Could you check a few things on this model? Use its own coordinates, in mm. Face numbers are marked on the shaded views. Coordinates: 2 decimals unless noted, no trailing zeros. Order: outer loops, then holes, each group sorted by start corner. A loop starts at its lowest first (then second) coordinate and runs counter-clockwise, first axis right, second up. Notation, with made-up numbers: (9.5, 43) - (23.5, 43) arc R14 ccw to (23.5, 69) - close; hole circle Ø8 at (24, -6.5). An arc over 180 degrees is marked (long way). One line per item, written item: value.
from build123d import *

# Parameters (mm, degrees)
F2_DEPTH = 12.7
F1_R     = 6.35
F3_DEPTH = 25.4


with BuildPart() as f2:
    # F0 (on Front) → F2 (new body)
    with BuildSketch(Plane.XZ):
        with BuildLine():
            ThreePointArc((-28.403627, 25.393778), (-36.341802, -10.856114), (-9.82124, -36.812406))
            Line((-9.82124, -36.812406), (-3.273747, -12.270802))
            ThreePointArc((-3.273747, -12.270802), (17.211851, -4.772017), (20.836528, 16.739681))
            ThreePointArc((20.836528, 16.739681), (-1.537184, 33.848118), (-28.403627, 25.393778))
        make_face()
    extrude(amount=F2_DEPTH)

    # F1 (on face) → F3 (cut)
    with BuildSketch(Plane.XZ):
        Circle(F1_R)
    extrude(amount=F3_DEPTH, mode=Mode.SUBTRACT)


solid = f2.part
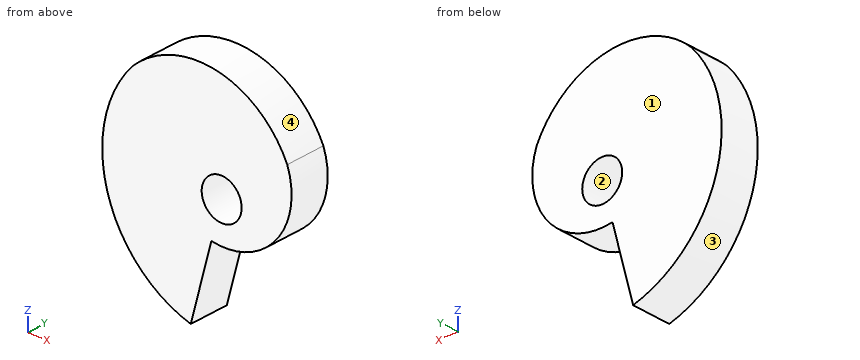
Item 1: I want a section at D-D on x = -20. Please give me the cut outline in (y, z).
Conclusion:
outline: (-12.7, -32.33) - (0, -32.33) - (0, 31.33) - (-12.7, 31.33) - close
Item 2: I want a section at A-A on x = 0. Please give me the cut outline in (y, z).
Conclusion:
outline: (-12.7, -12.6) - (0, -12.6) - (0, -6.35) - (-12.7, -6.35) - close; (-12.7, 6.35) - (0, 6.35) - (0, 33.54) - (-12.7, 33.54) - close
Item 3: If I drill on probe 1 along Z at (x, y) = (0, -9.5); probe 2 along X at (y, z) = (-2.5, 0); probe 3 along Z at (x, y) = (5, -3.5), over which ranges is the centre line in solid material (lowest first)?
Conclusion:
probe 1: -12.6 to -6.35, 6.35 to 33.54
probe 2: -37.94 to -6.35, 6.35 to 20.22
probe 3: -12.14 to -3.91, 3.91 to 31.93
Item 4: Thinking about a two-plate mould opening in X: for the marked faces 1, 2, 3 and 4, which applies, pulls with the +X half, pulls with the -X half, needs draft (parallel to the pull), parting line crosses it, or undercut?
Conclusion:
face 1: needs draft
face 2: undercut
face 3: pulls with the -X half
face 4: parting line crosses it
Item 5: I want a section at C-C on y = -9.25. Please give me the cut outline in (x, z), then the cut area to 3 significant figures.
Conclusion:
outline: (-28.4, 25.39) arc R38.29 ccw to (-9.82, -36.81) - (-3.27, -12.27) arc R21.71 ccw to (20.84, 16.74) arc R30.56 ccw to start; hole circle Ø12.7 at (0, 0)
area: 2,700 mm²
Item 6: I want a section at B-B on z = 2.5. Please give me the cut outline in (x, y), then the cut area to 3 significant figures.
Conclusion:
outline: (-37.87, -12.7) - (-5.84, -12.7) - (-5.84, 0) - (-37.87, 0) - close; (5.84, -12.7) - (21.2, -12.7) - (21.2, 0) - (5.84, 0) - close
area: 602 mm²
Item 7: I'm going to push flat-ended pins straight in: pin 1 Ø1 at (x, y) = (-28, -10.5) entering from -Z; pin 2 Ø1 at (y, z) = (-6, -28) entering from -X. Where does each tip first touch, or does it pass through?
Conclusion:
pin 1: z = -26.18
pin 2: x = -26.19
